Autodesk Inventor part; units mm, degrees
ref_plane "Work Plane1" through (0, 0, 0) normal (0, 0, 1) x (1, 0, 0)
ref_plane "YZ Plane" through (0, 0, 0) normal (1, 0, 0) x (0, 1, 0)
ref_plane "XZ Plane" through (0, 0, 0) normal (0, 1, 0) x (-1, 0, 0)
ref_plane "Work Plane1" through (0, 0, 0) normal (0, 0, 1) x (1, 0, 0)
sketch "Sketch1" plane through (0, 0, 0) normal (0, 0, 1) x (1, 0, 0)
  line L0 (300, -173.2051) -> (0, -346.4102)
  line L1 (0, -346.4102) -> (-300, -173.2051)
  line L2 (-300, -173.2051) -> (-300, 173.2051)
  line L3 (-300, 173.2051) -> (0, 346.4102)
  line L4 (0, 346.4102) -> (300, 173.2051)
  line L5 (300, 173.2051) -> (300, -173.2051)
  point P0 (0, 0)
  point P1 (0, 0)
  dimension "d0" = 300
extrude "Extrusion1" add sketch "Sketch1" along normal blind 60
properties part number "Gel" material "Phenolic Resin"
Could you check a few things on this model? Use its own coordinates, in mm. Give positions to 0.01 mm unless a question says otherwise; leave off trailing zeros. Order: outer loops, then holes, each group sorted by start corner. A loop starts at its lowest first (then second) coordinate and runs counter-clockwise, first axis right, second up. Notation, with made-up numbers: (72, 67) -> (104, 67) arc R32 cw to (104, 97) -> close; hole circle Ø1 at (21, 28). An arc over 180 degrees is marked (long way). Return JSON: item names as keys, results as strings.
1. Imagine slicing it at B-B on y = 188.5. List the corners of the cut face in (x, z) for me, then the cut area to 3 significant figures.
Answer list:
{"outline": "(-273.51, 0) -> (273.51, 0) -> (273.51, 60) -> (-273.51, 60) -> close", "area": "32,800 mm2"}
2. Imagine slicing it at C-C on x = -135. List the corners of the cut face in (y, z) for me, then the cut area to 3 significant figures.
Answer list:
{"outline": "(-268.47, 0) -> (268.47, 0) -> (268.47, 60) -> (-268.47, 60) -> close", "area": "32,200 mm2"}
3. Imagine slicing it at A-A on z = 45. List the corners of the cut face in (x, y) for me, then the cut area to 3 significant figures.
Answer list:
{"outline": "(-300, -173.21) -> (0, -346.41) -> (300, -173.21) -> (300, 173.21) -> (0, 346.41) -> (-300, 173.21) -> close", "area": "312,000 mm2"}
4. I need wall thicknesses on line 1 (Y direction, x = 80.5, z = 49); line 2 (Y direction, x = -148, z = 57); line 3 (X direction, y = -230, z = 14). Which ranges of each line are inside material? Lowest first, please. Write a range as from..to.
Answer list:
{"line 1": "y = -299.93..299.93", "line 2": "y = -260.96..260.96", "line 3": "x = -201.63..201.63"}
5. For pin 1 Ø6 at (x, z) = (71.5, 49) entering from +Y; pin 2 Ø6 at (x, z) = (158, 31) entering from +Y; pin 3 Ø1.5 at (x, y) = (-183, 226.5) entering from -Z; pin 4 Ø6 at (x, z) = (95, 30.5) entering from +Y, each with a flat end and sliding along its axis, tell me the tip position at first contact or that it passes through.
Answer list:
{"pin 1": "stops at y = 306.86", "pin 2": "stops at y = 256.92", "pin 3": "stops at z = 0", "pin 4": "stops at y = 293.29"}
